For this review, take the finished solid that the model builds, in its own axes (mm). Coordinates: 2 decimals unless noted, no trailing zeros. Order: outer loops, then holes, each group sorted by start corner. A loop starts at its lowest first (then second) coordinate and runs counter-clockwise, first axis right, second up. Notation, with made-up numbers: (67.5, -39.5) -> (93.5, -39.5) arc R24 ccw to (93.5, -19.5) -> close; hole circle Ø7 at (-27.5, 16). An arc over 180 degrees is marked (long way). Return JSON: item names as keys, results as strings. Group by question number.
Item 1: Take a section at A-A (z = 0). Write out the cut boundary in (x, y).
Item 2: Take a section at B-B (y = 6). Write out the cut boundary in (x, z), then the cut area to 3 significant figures.
Item 3: Insertion check: pin 1 (1.5 mm diameter, centred on x = -177, z = -26.5, fed in from -Y); pin 2 (1 mm diameter, centred on x = -29, y = 1.5, fed in from -Z); pin 3 (4 mm diameter, centred on x = 25, y = 5, fed in from +Z). Each pin has a flat end and moves straight along its axis. Give the tip position at first contact, or say it passes through.
Item 4: Draft analysis for pull direction X (two halves, no side actions). For faces 1 (the flat face through (-225, 5, -2)), 2 (the cylindrical face through (54.99, 4.93, 0.98)), 3 (the flat face through (-198, 5, 110)), 4 (the cylindrical face through (-24.397, 4.93, 12.69)), state which applies: +X half, -X half, draft (parallel to the pull), parting line (faces both ways), or undercut.
Item 5: For line 1 along X through (y, z) = (7, 0); line 2 along X through (y, z) = (1.5, 14); line 3 along Z through (x, y) = (-14.5, 4.75), list the stretches that pass through material, from the lowest coordinate up.
Item 6: Take a section at C-C (x = 0). Write out the cut boundary in (y, z), then the cut area to 3 significant figures.
Item 7: Take a section at D-D (x = -153). Write out the cut boundary in (y, z).
```python
from build123d import *

# Parameters (mm, degrees)
SKETCH_W_DIMENSIONS_R = 27.5
EXTRUDE_10MM_DEPTH    = 10


with BuildPart() as part:
    # sketch_w_dimensions → extrude_10mm (new body)
    with BuildSketch(Plane(origin=(0, 0, 0), x_dir=(1, 0, 0), z_dir=(0, 1, 0))):
        with BuildLine():
            Line((-225, 110), (-225, -110))
            Line((-225, -110), (-170, -110))
            Line((-170, -110), (16.21278302, -52.556119213))
            ThreePointArc((16.21278302, -52.556119213), (55, 0), (16.21278302, 52.556119213))
            Line((16.21278302, 52.556119213), (-170, 110))
            Line((-170, 110), (-225, 110))
        make_face()
        with Locations(Location((0, 0, 0), (0, 0, 270))):
            Circle(SKETCH_W_DIMENSIONS_R, mode=Mode.SUBTRACT)
    extrude(amount=EXTRUDE_10MM_DEPTH)


solid = part.part
```
Findings below:
{
 "1": {"outline": "(-225, 0) -> (-27.5, 0) -> (-27.5, 10) -> (-225, 10) -> close; (27.5, 0) -> (55, 0) -> (55, 10) -> (27.5, 10) -> close"},
 "2": {"outline": "(-225, -110) -> (-170, -110) -> (16.21, -52.56) arc R55 ccw to (16.21, 52.56) -> (-170, 110) -> (-225, 110) -> close; hole circle Ø55 at (0, 0)", "area": "43,000 mm2"},
 "3": {"pin 1": "stops at y = 0", "pin 2": "stops at z = -66.66", "pin 3": "stops at z = 49.96"},
 "4": {"face 1": "-X half", "face 2": "+X half", "face 3": "draft", "face 4": "undercut"},
 "5": {"line 1": "x = -225 to -27.5, 27.5 to 55", "line 2": "x = -225 to -23.67, 23.67 to 53.19", "line 3": "z = -62.03 to -23.37, 23.37 to 62.03"},
 "6": {"outline": "(0, -57.56) -> (10, -57.56) -> (10, -27.5) -> (0, -27.5) -> close; (0, 27.5) -> (10, 27.5) -> (10, 57.56) -> (0, 57.56) -> close", "area": "601 mm2"},
 "7": {"outline": "(0, -104.76) -> (10, -104.76) -> (10, 104.76) -> (0, 104.76) -> close"}
}
